from build123d import *

# Parameters (mm, degrees)
FILLET1_R = 0.25


with BuildPart() as part:
    # Sketch1 → Revolve1 (revolve)
    with BuildSketch(Plane(origin=(0, 0, 0), x_dir=(-1, 0, 0), z_dir=(0, 1, 0))):
        Polygon((-5, 1), (-7.5, 1), (-7.5, 0), (-4, 0), (-4, 15), (-4.711324865, 15), (-5, 14.5), align=None)
    revolve(axis=Axis((0, 0, 0), (0, 0, 1)))

    # Fillet1
    fillet1_edges = [part.edges().sort_by_distance(p)[0] for p in [
        (-5, 0, 1),
    ]]
    fillet(fillet1_edges, radius=FILLET1_R)


solid = part.part
The model under review builds one solid part; all positions refer to its coordinate system, in mm. A direction names the side the tool comes from. Give positions to 0.01 mm unless a question says otherwise; leave off trailing zeros. Order: outer loops, then holes, each group sorted by start corner. A loop starts at its lowest first (then second) coordinate and runs counter-clockwise, first axis right, second up. Notation, with made-up numbers: M 20.5,76 L 58.5,76 A29 ccw 58.5,103 Z; hole C 80.5,-20 d3. An arc over 180 degrees is marked long. One line per question, with ' | ' between items. Start each with the question number.
1) Wall thickness on L1, parallel to Y at x = 0, z = 8; L2, parallel to Z at x = -6, y = 0.5; L3, parallel to Y at x = -3.5, z = 3.5: over which ranges is each line inside the solid? List them lowest first. Write a range as from..to.
2) Mouldability with a two-part tool opening along X and no side actions: class faces 1 (the face through (-0.867, -3.905, 7.605)), 2 (the face through (-7.493, 0.33, 0.493)), 3 (the face through (4, -2, 15)) as pulls with the +X half, pulls with the -X half, needs draft (parallel to the pull), parting line crosses it, or undercut.
3) For faces 4 (the face through (3, -3, 0)), 5 (the face through (-1.08, -4.88, 7.78)), list the 3-axis set-ups (+Z, -Z, +X, -X, +Y, -Y) from which the entire face can be reached by the end or side of a thin tool; tool diameter is ignored.
4) Consider section A-A, the plane y = 0. Give the boundary of the cut face in (x, z), then the cut area to 3 significant figures.
5) Consider section D-D, the plane x = 5.75. Give the boundary of the cut face in (y, z).
6) Consider section C-C, the plane z = 11.75. Give the boundary of the cut face in (x, y).
7) Clearance check with flat-ended pins moving along their axes: P1, Ø1.5, axis at x = 3, z = 3, coming from the +Y side; P2, Ø3, axis at x = -1.5, y = -0.5, coming from the +Z side; P3, Ø6, axis at y = 4, z = 5.5, coming from the +X side; P4, Ø4, axis at x = -1.5, z = 2.5, coming from the +Y side. State where each tip first meets the part, or that it passes through.
Found:
1) L1: y = -5..-4, 4..5 | L2: z = 0..1 | L3: y = -3.57..-1.94, 1.94..3.57
2) face 1: undercut | face 2: parting line crosses it | face 3: needs draft
3) face 4: -Z, +X, -X, +Y, -Y | face 5: +Z
4) outline: M -7.5,0 L -4,0 L -4,15 L -4.71,15 L -5,14.5 L -5,1.25 A0.25 cw -5.25,1 L -7.5,1 Z; M 4,0 L 7.5,0 L 7.5,1 L 5.25,1 A0.25 cw 5,1.25 L 5,14.5 L 4.71,15 L 4,15 Z | area: 34.9 mm²
5) outline: M -4.82,0 L 4.82,0 L 4.82,1 L -4.82,1 Z
6) outline: C 0,0 d10; hole C 0,0 d8
7) P1: stops at y = 4.47 | P2: passes through | P3: stops at x = 4.9 | P4: stops at y = 7.5
